CAD build for the part. Positions are in the model's coordinates, mm. A direction names the side the tool comes from. Coordinates: 2 decimals unless noted, no trailing zeros. Order: outer loops, then holes, each group sorted by start corner. A loop starts at its lowest first (then second) coordinate and runs counter-clockwise, first axis right, second up. Notation, with made-up numbers: M 40,-6.5 L 93,-6.5 A23 ccw 93,32.5 Z; hole C 46.25,76.25 d9. An arc over 180 degrees is marked long. Write item = value, one per line.
from build123d import *

# Parameters (mm, degrees)
CROQUIS1_R              = 15
SALIENTE_EXTRUIR1_DEPTH = 18
SALIENTE_EXTRUIR2_DEPTH = 45
CROQUIS3_R              = 15
SALIENTE_EXTRUIR3_DEPTH = 20
REDONDEO1_R             = 10
REDONDEO2_R             = 10


with BuildPart() as part:
    # Croquis1 → Saliente-Extruir1 (new, symmetric)
    with BuildSketch(Plane(origin=(0, 0, 0), x_dir=(1, 0, 0), z_dir=(0, 1, 0))):
        with BuildLine():
            Line((24, 18), (67.5, 18))
            Line((67.5, 18), (67.5, -18))
            Line((67.5, -18), (24, -18))
            ThreePointArc((24, -18), (-30, 0), (24, 18))
        make_face()
        with Locations(Location((0, 0, 0), (0, 0, 270))):
            Circle(CROQUIS1_R, mode=Mode.SUBTRACT)
    extrude(amount=SALIENTE_EXTRUIR1_DEPTH, both=True)

    # Croquis2 → Saliente-Extruir2 (add)
    with BuildSketch(Plane(origin=(67.5, 0, 0), x_dir=(0, 0, -1), z_dir=(1, 0, 0))):
        Polygon((-18, 7.455844123), (-18, -7.455844123), (-7.455844123, -18), (7.455844123, -18), (18, -7.455844123), (18, 7.455844123), (7.455844123, 18), (-7.455844123, 18), align=None)
    extrude(amount=SALIENTE_EXTRUIR2_DEPTH)

    # Croquis3 → Saliente-Extruir3 (add)
    with BuildSketch(Plane(origin=(112.5, 0, 0), x_dir=(0, 0, -1), z_dir=(1, 0, 0))):
        Circle(CROQUIS3_R)
    extrude(amount=SALIENTE_EXTRUIR3_DEPTH)

    # Redondeo1
    # the kernel refuses this fillet: 10 mm, written as the material it adds along each edge
    with BuildSketch(Plane(origin=(67.5, 10.221825407, 35.67766953), x_dir=(1, 0, 0), z_dir=(0, -0.7071067811865474, -0.7071067811865477))) as redondeo1_piece_1_section:
        with BuildLine():
            CenterArc((REDONDEO1_R, REDONDEO1_R), REDONDEO1_R, 180, 90)
            Line((0, REDONDEO1_R), (0, 0))
            Line((0, 0), (REDONDEO1_R, 0))
        make_face()
    redondeo1_piece_1 = extrude(amount=64.911688245, mode=Mode.PRIVATE)
    redondeo1_piece_1 = split(redondeo1_piece_1, bisect_by=Plane(origin=(70.275136412, -18, 13.729156697), z_dir=(0, 1, 0)), keep=Keep.TOP, mode=Mode.PRIVATE)
    redondeo1_piece_1 = split(redondeo1_piece_1, bisect_by=Plane(origin=(70.275136412, -13.729156697, 18), z_dir=(0, 0, -1)), keep=Keep.TOP, mode=Mode.PRIVATE)
    add(redondeo1_piece_1)
    with BuildSketch(Plane(origin=(67.5, -35.67766953, 10.221825407), x_dir=(0, -0.7071067811865476, -0.7071067811865476), z_dir=(0, 0.7071067811865475, -0.7071067811865476))) as redondeo1_piece_2_section:
        with BuildLine():
            CenterArc((REDONDEO1_R, -REDONDEO1_R), REDONDEO1_R, 90, 90)
            Line((0, -REDONDEO1_R), (0, 0))
            Line((0, 0), (REDONDEO1_R, 0))
        make_face()
    redondeo1_piece_2 = extrude(amount=64.911688245, mode=Mode.PRIVATE)
    redondeo1_piece_2 = split(redondeo1_piece_2, bisect_by=Plane(origin=(70.275136413, -13.729156697, -18), z_dir=(0, 0, 1)), keep=Keep.TOP, mode=Mode.PRIVATE)
    redondeo1_piece_2 = split(redondeo1_piece_2, bisect_by=Plane(origin=(70.275136413, -18, -13.729156697), z_dir=(0, 1, 0)), keep=Keep.TOP, mode=Mode.PRIVATE)
    add(redondeo1_piece_2)
    with BuildSketch(Plane(origin=(67.5, -10.221825407, -35.67766953), x_dir=(1, 0, 0), z_dir=(0, 0.7071067811865477, 0.7071067811865474))) as redondeo1_piece_3_section:
        with BuildLine():
            CenterArc((REDONDEO1_R, REDONDEO1_R), REDONDEO1_R, 180, 90)
            Line((0, REDONDEO1_R), (0, 0))
            Line((0, 0), (REDONDEO1_R, 0))
        make_face()
    redondeo1_piece_3 = extrude(amount=64.911688245, mode=Mode.PRIVATE)
    redondeo1_piece_3 = split(redondeo1_piece_3, bisect_by=Plane(origin=(70.275136412, 13.729156697, -18), z_dir=(0, 0, 1)), keep=Keep.TOP, mode=Mode.PRIVATE)
    redondeo1_piece_3 = split(redondeo1_piece_3, bisect_by=Plane(origin=(70.275136412, 18, -13.729156697), z_dir=(0, -1, 0)), keep=Keep.TOP, mode=Mode.PRIVATE)
    add(redondeo1_piece_3)
    with BuildSketch(Plane(origin=(67.5, 35.67766953, -10.221825407), x_dir=(1, 0, 0), z_dir=(0, -0.7071067811865476, 0.7071067811865476))) as redondeo1_piece_4_section:
        with BuildLine():
            CenterArc((REDONDEO1_R, REDONDEO1_R), REDONDEO1_R, 180, 90)
            Line((0, REDONDEO1_R), (0, 0))
            Line((0, 0), (REDONDEO1_R, 0))
        make_face()
    redondeo1_piece_4 = extrude(amount=64.911688245, mode=Mode.PRIVATE)
    redondeo1_piece_4 = split(redondeo1_piece_4, bisect_by=Plane(origin=(70.275136412, 18, 13.729156697), z_dir=(0, -1, 0)), keep=Keep.TOP, mode=Mode.PRIVATE)
    redondeo1_piece_4 = split(redondeo1_piece_4, bisect_by=Plane(origin=(70.275136412, 13.729156697, 18), z_dir=(0, 0, -1)), keep=Keep.TOP, mode=Mode.PRIVATE)
    add(redondeo1_piece_4)

    # Redondeo2
    redondeo2_edges = [part.edges().sort_by_distance(p)[0] for p in [
        (24, 0, 18),
        (24, 0, -18),
    ]]
    fillet(redondeo2_edges, radius=REDONDEO2_R)


solid = part.part
(1) Tool access for faces 1 (the face through (61, 0, -18)), 2 (the face through (94.755, 12.802, 12.654)), 3 (the face through (94.755, -12.802, -12.654)), 4 (the face through (122.36, 0.66, 14.985)), 5 (the face through (94.755, -12.654, 12.802)): list every direction of +Z, -Z, +X, -X, +Y, -Y with a clear straight run to the whole face (end or side of a thin tool).
Evaluation:
face_1 = -Z, +X, +Y, -Y
face_2 = +Z, +X, +Y
face_3 = -Z, +X, -Y
face_4 = +X
face_5 = +Z, +X, -Y
(2) Slice it at B-B, the plane y = 0. Write the cut outline in (x, z), then the cut area to 3 significant figures.
Evaluation:
outline = M 21.42,-21 A10 cw 28.57,-18 L 112.5,-18 L 112.5,-15 L 132.5,-15 L 132.5,15 L 112.5,15 L 112.5,18 L 28.57,18 A10 cw 21.42,21 A30 ccw long Z; hole C 0,0 d30
area = 5,760 mm²
(3) Pull direction Y, two halves, no side cores. Call faces 6 (the face through (72.531, -13.589, 13.736)), 7 (the face through (72.531, 13.589, -13.736)), 8 (the face through (62, 0, 18)): +Y half, -Y half, draft (parallel to the pull), parting line (faces both ways), or undercut.
Evaluation:
face_6 = -Y half
face_7 = +Y half
face_8 = draft
(4) Wall check: line 1 (Z direction, x = 37.5, y = 13); line 2 (Z direction, x = -5, y = 9); line 3 (X direction, y = 4, z = 10). Give the ranges that are in metal, low to high. Write a range as from..to.
Evaluation:
line_1 = -18..18
line_2 = -29.58..-14.14, 14.14..29.58
line_3 = -28.28..-11.18, 11.18..132.5
(5) Slice it at D-D, the plane x = 85.5. Write the cut outline in (y, z).
Evaluation:
outline = M -18,-7.46 L -7.46,-18 L 7.46,-18 L 18,-7.46 L 18,7.46 L 7.46,18 L -7.46,18 L -18,7.46 Z
(6) Slice it at A-A, the plane z = 0. Write the cut outline in (x, y).
Evaluation:
outline = M -30,-18 L -15,-18 L -15,18 L -30,18 Z; M 15,-18 L 112.5,-18 L 112.5,-15 L 132.5,-15 L 132.5,15 L 112.5,15 L 112.5,18 L 15,18 Z
(7) Slice it at C-C, the plane x = 0. Write the cut outline in (y, z).
Evaluation:
outline = M -18,-30 L 18,-30 L 18,-15 L -18,-15 Z; M -18,15 L 18,15 L 18,30 L -18,30 Z
(8) Pin check, flat tips, straight feed: pin 1 Ø11 at (x, y) = (62.5, 2) entering from -Z; pin 2 Ø2 at (x, y) = (16.5, 2.5) entering from +Z; pin 3 Ø12 at (y, z) = (5.5, -8) entering from -X. Stop position of each tip, or through.
Evaluation:
pin_1 = -18
pin_2 = 25.69
pin_3 = -29.93
